Work out the finished part from the listing and answer in its coordinate system (mm). Face numbers are marked on the shaded views. A direction names the side the tool comes from. Give positions to 0.01 mm unless a question says otherwise; leave off trailing zeros. Loops run counter-clockwise (first coordinate to the right, second up) from the corner with the lowest first, then second, coordinate; pieces in that order, holes last. Notation, with made-up numbers: M 73,48 L 102,48 A12 cw 102,62 Z; hole C 39,71.5 d2. An arc over 180 degrees is marked long. Use a Markdown table: item, result.
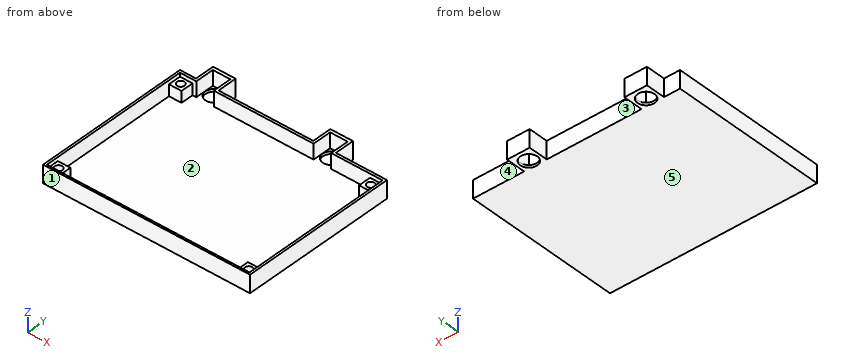
```python
from build123d import *

# Parameters (mm, degrees)
F0_W     = 82.5
F0_H     = 70
F1_DEPTH = 7
F2_W     = 7
F2_H     = 7.5
F3_DEPTH = 6
F4_R     = 3.375
F5_DEPTH = 25
F6_W     = 5
F6_H     = 5
F6_R     = 1.5
F7_DEPTH = 4.5
F8_W     = 6.375
F8_H     = 7.75
F8_W_2   = 37.75
F8_W_3   = 20.375
F9_DEPTH = 25


with BuildPart() as f1:
    # F0 (on Top) → F1 (new body)
    with BuildSketch(Plane.XY):
        Rectangle(F0_W, F0_H)
    extrude(amount=F1_DEPTH)

    # F2 (on face) → F3 (cut)
    with BuildSketch(Plane.XY.offset(7)):
        Polygon((40.375, -34.25), (40.375, 26.25), (19.875, 26.25), (12.875, 26.25), (-26.875, 26.25), (-33.875, 26.25), (-40.375, 26.25), (-40.375, -34.25), align=None)
        with Locations((-30.375, 30)):
            Rectangle(F2_W, F2_H)
        with Locations((16.375, 30)):
            Rectangle(F2_W, F2_H)
    extrude(amount=-F3_DEPTH, mode=Mode.SUBTRACT)

    # F4 (on face) → F5 (cut)
    with BuildSketch(Plane.XY.offset(1)):
        with Locations((-30.375, 30.25)):
            Circle(F4_R)
        with Locations((16.375, 30.25)):
            Circle(F4_R)
    extrude(amount=-F5_DEPTH, mode=Mode.SUBTRACT)

    # F6 (on face) → F7 (join)
    with BuildSketch(Plane.XY.offset(1)):
        with Locations((37.875, 23.75)):
            Rectangle(F6_W, F6_H)
        with Locations((37.875, 23.75)):
            Circle(F6_R, mode=Mode.SUBTRACT)
        with Locations((37.875, -31.75)):
            Rectangle(F6_W, F6_H)
        with Locations((37.875, -31.75)):
            Circle(F6_R, mode=Mode.SUBTRACT)
        with Locations((-37.875, -31.75)):
            Rectangle(F6_W, F6_H)
        with Locations((-37.875, -31.75)):
            Circle(F6_R, mode=Mode.SUBTRACT)
        Polygon((-35.375, 26.25), (-40.375, 26.25), (-40.375, 21.25), (-35.375, 21.25), (-35.375, 23.75), align=None)
        with Locations((-37.875, 23.75)):
            Circle(F6_R, mode=Mode.SUBTRACT)
    extrude(amount=F7_DEPTH)

    # F8 (on face) → F9 (cut)
    with BuildSketch(Plane.XY.offset(7)):
        with Locations((-38.0625, 31.125)):
            Rectangle(F8_W, F8_H)
        with Locations((-7, 31.125)):
            Rectangle(F8_W_2, F8_H)
        with Locations((31.0625, 31.125)):
            Rectangle(F8_W_3, F8_H)
    extrude(amount=-F9_DEPTH, mode=Mode.SUBTRACT)


solid = f1.part
```
(1) A cutting plane is placed at D-D (z = 2.25). Count the separate pieces of the cut face and the enclosed holes in it, and give its area (3 significant figures).
Entries:
| item | result |
|---|---|
| separate pieces | 1 |
| enclosed holes | 5 |
| area | 356 mm² |
(2) Given P1, Ø3, axis at y = 28.5, z = 3, coming from the +X side; P2, Ø1.5, axis at x = -38.5, y = -32, coming from the +Z side; P3, Ø3.5, axis at x = 33.5, z = 4, coming from the +Y side; P4, Ø4, axis at x = 37.875, y = 23.75, coming from the +Z side, each flat-ended and moving along its own axis, determine where each tip first touches the part or whether it passes through.
Entries:
| item | result |
|---|---|
| P1 | stops at x = 41.25 |
| P2 | stops at z = 1 |
| P3 | stops at y = 27.25 |
| P4 | stops at z = 5.5 |
(3) The mould has two halves that part along X. Classify the marked faces 1 and 2: released by +X, released by -X, zero draft, split by the parting line, or undercut.
Entries:
| item | result |
|---|---|
| face 1 | zero draft |
| face 2 | undercut |
(4) A cutting plane is placed at B-B (x = 11). Write down the section's boundary in (y, z), and give its area (4 significant figures).
Entries:
| item | result |
|---|---|
| outline | M -35,0 L 27.25,0 L 27.25,7 L 26.25,7 L 26.25,1 L -34.25,1 L -34.25,7 L -35,7 Z |
| area | 72.75 mm² |
(5) A cutting plane is placed at C-C (y = 7). Write down the section's boundary in (x, z) (3 decimals).
Entries:
| item | result |
|---|---|
| outline | M -41.25,0 L 41.25,0 L 41.25,7 L 40.375,7 L 40.375,1 L -40.375,1 L -40.375,7 L -41.25,7 Z |
(6) Consider probe 1 along X at (y, z) = (30.5, 2.25) (3 decimals); probe 2 along Y at (x, z) = (20, 4); probe 3 along Y at (x, z) = (-33, 1.25). Determine where each line is inside the solid, lowest interval first. Write a range as [from, to].
Entries:
| item | result |
|---|---|
| probe 1 | x = [-34.875, -33.875], [-26.875, -25.875], [11.875, 12.875], [19.875, 20.875] |
| probe 2 | y = [-35, -34.25], [26.25, 35] |
| probe 3 | y = [-35, -34.25], [33.75, 35] |
(7) A cutting plane is placed at A-A (y = 30.25). Write down the section's boundary in (x, z) (3 decimals).
Entries:
| item | result |
|---|---|
| outline | M -34.875,0 L -33.75,0 L -33.75,1 L -33.875,1 L -33.875,7 L -34.875,7 Z; M -27,0 L -25.875,0 L -25.875,7 L -26.875,7 L -26.875,1 L -27,1 Z; M 11.875,0 L 13,0 L 13,1 L 12.875,1 L 12.875,7 L 11.875,7 Z; M 19.75,0 L 20.875,0 L 20.875,7 L 19.875,7 L 19.875,1 L 19.75,1 Z |
(8) Which of the six approach directions +Z, -Z, +X, -X, +Y, -Y give full straight-line access (tool end or side, diameter ignored) to the marked faces 3, 4 and 5?
Entries:
| item | result |
|---|---|
| face 3 | +Z, -Z, +Y |
| face 4 | +Z, -Z, +X, +Y |
| face 5 | -Z, +X, -X, +Y, -Y |
